Check sheet for the modelled part. Datum: model origin and axes. Units: mm. Face numbers are marked on the shaded views. A direction names the side the tool comes from. Round coordinates to 2 decimals unless told otherwise and drop trailing zeros. Write each loop counter-clockwise with the first axis right and the second up, starting at its lowest first coordinate (ties: lowest second). Pieces come first, ordered by that corner, then holes. Notation, with made-up numbers: (-29, 45.5) -> (18, 45.5) arc R29 ccw to (18, 72.5) -> close; hole circle Ø3 at (-0.5, 84.25). An arc over 180 degrees is marked (long way). Put each result on its own line as item: value. Start each with the question number.
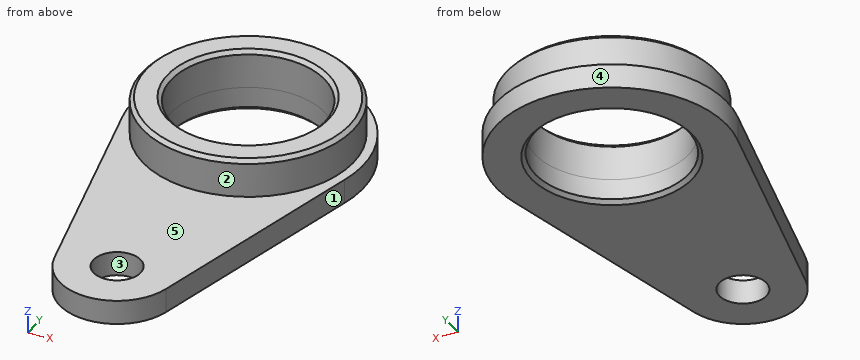
from build123d import *

# Parameters (mm, degrees)
CROQUIS1_R                          = 25
CROQUIS1_R_2                        = 6.15
SALIENTE_EXTRUIR1_DEPTH             = 6.35
CROQUIS2_R                          = 27.45
CROQUIS2_R_2                        = 20
SALIENTE_EXTRUIR2_DEPTH             = 10
SALIENTE_EXTRUIR2_DIRECTION_2_REACH = 87.676
CHAFL_N1_SIZE                       = 1


with BuildPart() as part:
    # Croquis1 → Saliente-Extruir1 (new body)
    with BuildSketch(Plane.XY):
        with BuildLine():
            Line((14.595331362, -68.460679477), (29.078013405, -7.380320889))
            ThreePointArc((29.078013405, -7.380320889), (0, 30), (-29.078013405, -7.380320889))
            Line((-29.078013405, -7.380320889), (-14.595331362, -68.460679477))
            ThreePointArc((-14.595331362, -68.460679477), (0, -80), (14.595331362, -68.460679477))
        make_face()
        Circle(CROQUIS1_R, mode=Mode.SUBTRACT)
        with Locations((0, -65)):
            Circle(CROQUIS1_R_2, mode=Mode.SUBTRACT)
    extrude(amount=SALIENTE_EXTRUIR1_DEPTH)

    # Croquis2 → Saliente-Extruir2 (add)
    with BuildSketch(Plane.XY.offset(6.35)):
        Circle(CROQUIS2_R)
        Circle(CROQUIS2_R_2, mode=Mode.SUBTRACT)
    extrude(amount=SALIENTE_EXTRUIR2_DEPTH)

    # Saliente-Extruir2 direction 2: up to this face of the body (flat: up to its plane)
    saliente_extruir2_direction_2_end = Plane(part.part.faces().sort_by_distance((0, -32.142670277, 0))[0])
    # Croquis2 → Saliente-Extruir2 direction 2 (add, up to the picked face)
    with BuildSketch(Plane.XY.offset(6.35), mode=Mode.PRIVATE) as saliente_extruir2_direction_2_sk1:
        Circle(CROQUIS2_R)
        Circle(CROQUIS2_R_2, mode=Mode.SUBTRACT)
    saliente_extruir2_direction_2_tool1 = split(extrude(saliente_extruir2_direction_2_sk1.sketch, amount=-SALIENTE_EXTRUIR2_DIRECTION_2_REACH, mode=Mode.PRIVATE), bisect_by=saliente_extruir2_direction_2_end, keep=Keep.BOTH, mode=Mode.PRIVATE)
    add(saliente_extruir2_direction_2_tool1.solids().sort_by(Axis((-26.673597, 0, 6.35), (0, 0, -1)))[0])

    # Chaflán1
    chafl_n1_edges = [part.edges().sort_by_distance(p)[0] for p in [
        (-20, 0, 0),
        (-20, 0, 16.35),
        (-27.45, 0, 16.35),
    ]]
    chamfer(chafl_n1_edges, length=CHAFL_N1_SIZE)


solid = part.part
1. Section check C-C, the plane z = 5.25. Enter the section's corners in (x, y), then the cut area to 3 significant figures.
2. Material ranges on L1, parallel to Y at x = 0, z = 2; L2, parallel to Y at x = 0, z = 12; L3, parallel to Z at x = 8.5, y = -36, recorded low to high. Write a range as [from, to].
3. Gauge pin test, flat ends, axial feed: P1, Ø8, axis at x = -8.5, z = 2, coming from the -Y side; P2, Ø10, axis at x = 7.5, y = 7, coming from the +Z side; P3, Ø6, axis at x = 17.5, z = 10.5, coming from the +Y side; P4, Ø6, axis at x = 16.5, z = 2.5, coming from the -Y side. Record the tip position at first contact, or that the pin passes through.
4. Access from +Z, -Z, +X, -X, +Y, -Y to the whole of each face (thin tool, end or side, straight path). Record for the marked faces 1 and 2.
5. Section check B-B, the plane y = 0. Enter the section's corners in (x, z).
6. Draft check along X on the marked faces 3, 4 and 5. Enter one of: released by +X, released by -X, zero draft, split by the parting line, or undercut.
7. Section check D-D, the plane z = 11. Enter the section's corners in (x, y), then the cut area to 3 significant figures.
8. Section check A-A, the plane x = 0. Enter the section's corners in (y, z), then the cut area to 3 significant figures.
Reply:
1. outline: (-29.08, -7.38) -> (-14.6, -68.46) arc R15 ccw to (14.6, -68.46) -> (29.08, -7.38) arc R30 ccw (long way) to start; hole circle Ø40 at (0, 0); hole circle Ø12.3 at (0, -65)
1. area: 3,390 mm2
2. L1: y = [-80, -71.15], [-58.85, -20], [20, 30]
2. L2: y = [-27.45, -20], [20, 27.45]
2. L3: z = [0, 6.35]
3. P1: stops at y = -79.31
3. P2: passes through
3. P3: stops at y = 23.31
3. P4: stops at y = -71.54
4. face 1: +Z, -Z, +X, -Y
4. face 2: +Z
5. outline: (-30, 0) -> (-21, 0) -> (-20, 1) -> (-20, 15.35) -> (-21, 16.35) -> (-26.45, 16.35) -> (-27.45, 15.35) -> (-27.45, 6.35) -> (-30, 6.35) -> close; (20, 1) -> (21, 0) -> (30, 0) -> (30, 6.35) -> (27.45, 6.35) -> (27.45, 15.35) -> (26.45, 16.35) -> (21, 16.35) -> (20, 15.35) -> close
6. face 3: undercut
6. face 4: split by the parting line
6. face 5: zero draft
7. outline: circle Ø54.9 at (0, 0); hole circle Ø40 at (0, 0)
7. area: 1,110 mm2
8. outline: (-80, 0) -> (-71.15, 0) -> (-71.15, 6.35) -> (-80, 6.35) -> close; (-58.85, 0) -> (-21, 0) -> (-20, 1) -> (-20, 15.35) -> (-21, 16.35) -> (-26.45, 16.35) -> (-27.45, 15.35) -> (-27.45, 6.35) -> (-58.85, 6.35) -> close; (20, 1) -> (21, 0) -> (30, 0) -> (30, 6.35) -> (27.45, 6.35) -> (27.45, 15.35) -> (26.45, 16.35) -> (21, 16.35) -> (20, 15.35) -> close
8. area: 512 mm2
